```python
from build123d import *

# Parameters (mm, degrees)
CROQUIS1_W                      = 1100
CROQUIS1_H                      = 220
BRIDA_BASE1_DEPTH               = 1.5
PLIEGUE_START                   = -592.530487805
PLIEGUE_CROQUIZADO1_DEPTH       = 1100
PLIEGUE_CROQUIZADO1_2_OUTLINE_W = 55.321902755
PLIEGUE_CROQUIZADO1_2_OUTLINE_H = 1.5
PLIEGUE_CROQUIZADO1_2_DEPTH     = 1100
CROQUIS8_R                      = 3
CORTAR_EXTRUIR1_DEPTH           = 10
TALADRO_DE_MARGEN_PARA_M51_D    = 5.5


# Read off the part's stored shape, not the designer's step: Pliegue croquizado1
# Sheet-metal steps are written as plain solids
with BuildPart() as part:
    # Croquis1 → Brida base1 (new body)
    with BuildSketch(Plane(origin=(0, 0, 0), x_dir=(1, 0, 0), z_dir=(0, 1, 0))):
        with Locations((-42.530487805, -13.391768293)):
            Rectangle(CROQUIS1_W, CROQUIS1_H)
    extrude(amount=-BRIDA_BASE1_DEPTH)

    # Pliegue croquizado1 outline → Pliegue croquizado1 (cut)
    with BuildSketch(Plane.YZ.offset(PLIEGUE_START)):
        with BuildLine():
            Line((0, -96.608231707), (0, -41.608231707))
            ThreePointArc((0, -41.608231707), (-1.060660172, -41.168891879), (-1.5, -40.108231707))
            Line((-1.5, -40.108231707), (-1.5, -96.608231707))
            Line((-1.5, -96.608231707), (0, -96.608231707))
        make_face()
        with BuildLine():
            Line((-1.5, 123.391768293), (-1.5, 66.891768293))
            ThreePointArc((-1.5, 66.891768293), (-1.060660171, 67.952428465), (0, 68.391768293))
            Line((0, 68.391768293), (0, 123.391768293))
            Line((0, 123.391768293), (-1.5, 123.391768293))
        make_face()
    extrude(amount=PLIEGUE_CROQUIZADO1_DEPTH, mode=Mode.SUBTRACT)

    # Pliegue croquizado1 2 outline → Pliegue croquizado1 2 (add)
    with BuildSketch(Plane.YZ.offset(PLIEGUE_START)):
        with Locations((27.660951378, -40.858231707)):
            Rectangle(PLIEGUE_CROQUIZADO1_2_OUTLINE_W, PLIEGUE_CROQUIZADO1_2_OUTLINE_H)
        with Locations((27.660951378, 67.641768293)):
            Rectangle(PLIEGUE_CROQUIZADO1_2_OUTLINE_W, PLIEGUE_CROQUIZADO1_2_OUTLINE_H)
    extrude(amount=PLIEGUE_CROQUIZADO1_2_DEPTH)

    # Croquis8 → Cortar-Extruir1 (cut)
    with BuildSketch(Plane(origin=(0, 0, 0), x_dir=(1, 0, 0), z_dir=(0, 1, 0))):
        with Locations(Location((-564.580402517, -56.391768293, 0), (0, 0, 270))):
            Circle(CROQUIS8_R)
        with Locations(Location((-540.580402517, -56.391768293, 0), (0, 0, 270))):
            Circle(CROQUIS8_R)
        with Locations(Location((-540.580402517, 29.608231707, 0), (0, 0, 270))):
            Circle(CROQUIS8_R)
        with Locations(Location((-564.580402517, 29.608231707, 0), (0, 0, 270))):
            Circle(CROQUIS8_R)
    extrude(amount=-CORTAR_EXTRUIR1_DEPTH, mode=Mode.SUBTRACT)

    # Taladro de margen para M51 (through all)
    with Locations(Plane(origin=(0, 0, 0), x_dir=(1, 0, 0), z_dir=(0, 1, 0))):
        with Locations((-512.530487805, -43.391768293), (-512.530487805, 16.608231707), (-112.530487805, -43.391768293), (-112.530487805, 16.608231707), (287.469512195, -43.391768293), (287.469512195, 16.608231707)):
            Hole(TALADRO_DE_MARGEN_PARA_M51_D / 2)


solid = part.part
```
Check sheet for the modelled part. Datum: model origin and axes. Units: mm. A direction names the side the tool comes from. Round coordinates to 2 decimals unless told otherwise and drop trailing zeros. Order: outer loops, then holes, each group sorted by start corner. A loop starts at its lowest first (then second) coordinate and runs counter-clockwise, first axis right, second up.
1) Scan lines: line 1 (Z direction, x = -324.5, y = 33); line 2 (Y direction, x = -468, z = -3). Record each from-to range of solid material in increasing order.
2) Section check A-A (y = 33). Record the boundary of the cut face in (x, z), and give its area (3 significant figures).
3) Mould release check, pull along Z, two halves, no side actions. Record for faces 1 (the flat face through (-50, 27, -41.608)), 2 (the flat face through (-50, 0, 13)), 3 (the flat face through (-50, 27, 68.392)): +Z half, -Z half, draft (parallel to the pull), parting line (faces both ways), or undercut.
4) Section check C-C (z = -2.5). Record the boundary of the cut face in (x, y), and give its area (3 significant figures).
5) Section check B-B (x = -524.5). Record the boundary of the cut face in (y, z), and give its area (3 significant figures).
6) Go/stop test with a flat-tipped pin: pin 1 Ø9 at (x, z) = (287.47, 43.39) entering from +Y. Record where the tip stops, or that it passes through.
7) Tool access check on faces 4 (the flat face through (-592.53, -1, 14)), 5 (the flat face through (-50, 27, 66.892)). Record the directions out of +Z, -Z, +X, -X, +Y, -Y that give a thin tool (end or side, any length) a straight path to the whole face; none if there is none.
Result:
1. line 1: z = -41.61 to -40.11, 66.89 to 68.39
1. line 2: y = -1.5 to 0
2. outline: (-592.53, -41.61) - (507.47, -41.61) - (507.47, -40.11) - (-592.53, -40.11) - close; (-592.53, 66.89) - (507.47, 66.89) - (507.47, 68.39) - (-592.53, 68.39) - close
2. area: 3,300 mm2
3. face 1: -Z half
3. face 2: undercut
3. face 3: +Z half
4. outline: (-592.53, -1.5) - (507.47, -1.5) - (507.47, 0) - (-592.53, 0) - close
4. area: 1,650 mm2
5. outline: (-1.5, -40.11) arc R1.5 ccw to (0, -41.61) - (55.32, -41.61) - (55.32, -40.11) - (0, -40.11) - (0, 66.89) - (55.32, 66.89) - (55.32, 68.39) - (0, 68.39) arc R1.5 ccw to (-1.5, 66.89) - close
5. area: 330 mm2
6. pin 1: stops at y = 0
7. face 4: +Z, -Z, -X, +Y, -Y
7. face 5: +X, -X, +Y
